Solid Edge part; units mm, degrees
sketch "Sketch1" plane through (0, 0, 0) normal (0, -1, 0) x (1, 0, 0)
  line L0 (-3.35, 1.1) -> (3.35, 1.1)
  line L1 (3.35, 0.6) -> (3.35, 1.1)
  line L2 (3.67, 0.6) -> (3.35, 0.6)
  line L3 (3.67, 0.25) -> (3.67, 0.6)
  line L4 (3.67, 0.25) -> (3.67, -0.1)
  line L5 (3.67, -0.1) -> (3.35, -0.1)
  line L6 (3.35, -0.1) -> (3.35, -1.1)
  line L7 (-3.35, -1.1) -> (3.35, -1.1)
  line L8 (-3.35, -0.1) -> (-3.35, -1.1)
  line L9 (-3.67, -0.1) -> (-3.35, -0.1)
  line L10 (-3.67, 0.25) -> (-3.67, -0.1)
  line L11 (-3.67, 0.25) -> (-3.67, 0.6)
  line L12 (-3.67, 0.6) -> (-3.35, 0.6)
  line L13 (-3.35, 0.6) -> (-3.35, 1.1)
extrude "Protrusion1" add sketch "Sketch1" against normal blind 3.5
sketch "Sketch2" plane through (0, 0, 0) normal (0, -1, 0) x (1, 0, 0)
  line L0 (2.95, 0.8) -> (-2.95, 0.8)
  line L1 (-2.95, 0.8) -> (-2.95, -0.8)
  line L2 (-2.95, -0.8) -> (2.95, -0.8)
  line L3 (2.95, -0.8) -> (2.95, 0.8)
extrude "BackSide_Hole_Cutout" cut sketch "Sketch2" against normal blind 0.2
sketch "Sketch3" plane through (0, 3.5, 0) normal (0, 1, 0) x (-1, 0, 0)
  line L0 (-2.45, 0.15) -> (-2.45, 0.35)
  line L1 (-2.45, 0.35) -> (-2.55, 0.35)
  line L2 (-2.55, 0.35) -> (-2.55, 0.15)
  line L3 (-2.55, 0.15) -> (-2.45, 0.15)
extrude "Pin_Cutout_Instance" cut sketch "Sketch3" against normal blind 2.3
chamfer "Chamfered_Edges" distance 0.2 angle 45 24 edges at (3.67, 3.5, 0.25) (-3.67, 3.5, 0.25) (-3.35, 3.5, 0.85) (3.35, 3.5, 0.85) (3.35, 3.5, -0.6) (0, 3.5, -1.1) (0, 3.5, 1.1) (3.51, 3.5, 0.6) (3.51, 3.5, -0.1) (-3.35, 3.5, -0.6) (-3.51, 3.5, -0.1) (-3.51, 3.5, 0.6) (3.35, 0, -0.6) (3.67, 0, 0.25) (3.35, 0, 0.85) (-3.35, 0, -0.6) (-3.67, 0, 0.25) (-3.35, 0, 0.85) (-3.51, 0, -0.1) (-3.51, 0, 0.6) (3.51, 0, 0.6) (3.51, 0, -0.1) (0, 0, 1.1) (0, 0, -1.1)
fillet "Round_Edges_Pin_Hole" radius 0.05 4 edges at (2.5, 3.5, 0.15) (2.45, 3.5, 0.25) (2.55, 3.5, 0.25) (2.5, 3.5, 0.35)
pattern_linear "Pattern1" count 6 spacing 1 along (-1, 0, 0) of "Pin_Cutout_Instance", "Round_Edges_Pin_Hole"
sketch "Sketch4" plane through (0, 0.2, 0) normal (0, -1, 0) x (1, 0, 0)
  circle A0 centre (-2.5, 0.25) radius 0.4
  circle A1 centre (-1.5, 0.25) radius 0.4
  circle A2 centre (-0.5, 0.25) radius 0.4
  circle A3 centre (0.5, 0.25) radius 0.4
  circle A4 centre (1.5, 0.25) radius 0.4
  circle A5 centre (2.5, 0.25) radius 0.4
extrude "Cable_Endings_Protruded" add sketch "Sketch4" along normal blind 0.2
properties material "ABS Plastic, high impact"
CAD build for the part. Positions are in the model's coordinates, mm. A direction names the side the tool comes from. Coordinates: 2 decimals unless noted, no trailing zeros. Write each loop counter-clockwise with the first axis right and the second up, starting at its lowest first coordinate (ties: lowest second). Pieces come first, ordered by that corner, then holes. Notation, with made-up numbers: (20, 37) -> (66, 37) arc R11 cw to (66, 43) -> close; hole circle Ø6 at (86.5, 87). An arc over 180 degrees is marked (long way). Return JSON: item names as keys, results as strings. Group by question number.
Q1. Cut at D-D, the plane y = 2.45. State how many separate pieces and enclosed holes the cut face has, then the cut area to 3 significant figures.
Q2. Pull direction Z, two halves, no side cores. Call faces 1 (the face through (0, 2, 1.1)), 2 (the face through (0, 0.2, 0)), 3 (the face through (0, 2, -1.1)), 4 (the face through (0, 3.5, 0)): released by +Z, released by -Z, zero draft, split by the parting line, or undercut.
Q3. Which spindle directions (+Z, -Z, +X, -X, +Y, -Y) get a long thin tool onto all of the face, cutting with end or side? Do faces 5 (the face through (-3.35, 1.7, -0.6)), 6 (the face through (3.35, 1.7, -0.6)). Say none if no direction does.
Q4. Flat gauge pin, fed straight in: pin 1 (0.8 mm diameter, centred on y = 1.5, z = -1, fed in from +X). Where does the tip first touch, or does it go through?
Q5. Cut at C-C, the plane x = -2.25. Give the cut face in (y, z).
Q6. Cut at B-B, the plane y = 0.5. Give the cut face in (x, z), then the cut area to 3 significant figures.
Q7. Drill centre lines: line 1 (Z direction, x = -1.5, y = 2.55); line 2 (Y direction, x = -0.5, z = 0.2); line 3 (Y direction, x = 0.25, z = 0.6). Where is each one in solid material? Low to high.
Q8. Cut at A-A, the plane z = -0.4. Give the cut face in (x, y).
Returned:
{
 "1": {"separate pieces": "1", "enclosed holes": "6", "area": "15.1 mm2"},
 "2": {"face 1": "released by +Z", "face 2": "undercut", "face 3": "released by -Z", "face 4": "zero draft"},
 "3": {"face 5": "-Z, -X, +Y, -Y", "face 6": "-Z, +X, +Y, -Y"},
 "4": {"pin 1": "stops at x = 3.35"},
 "5": {"outline": "(0, -0.9) -> (0.2, -1.1) -> (3.3, -1.1) -> (3.5, -0.9) -> (3.5, 0.9) -> (3.3, 1.1) -> (0.2, 1.1) -> (0, 0.9) -> (0, 0.8) -> (0.2, 0.8) -> (0.2, 0.56) -> (0, 0.56) -> (0, -0.06) -> (0.2, -0.06) -> (0.2, -0.8) -> (0, -0.8) -> close"},
 "6": {"outline": "(-3.67, -0.1) -> (-3.35, -0.1) -> (-3.35, -1.1) -> (3.35, -1.1) -> (3.35, -0.1) -> (3.67, -0.1) -> (3.67, 0.6) -> (3.35, 0.6) -> (3.35, 1.1) -> (-3.35, 1.1) -> (-3.35, 0.6) -> (-3.67, 0.6) -> close", "area": "15.2 mm2"},
 "7": {"line 1": "z = -1.1 to 0.15, 0.35 to 1.1", "line 2": "y = 0 to 1.2", "line 3": "y = 0.2 to 3.5"},
 "8": {"outline": "(-3.35, 0.2) -> (-3.15, 0) -> (-2.95, 0) -> (-2.95, 0.2) -> (2.95, 0.2) -> (2.95, 0) -> (3.15, 0) -> (3.35, 0.2) -> (3.35, 3.3) -> (3.15, 3.5) -> (-3.15, 3.5) -> (-3.35, 3.3) -> close"}
}
